Autodesk Inventor part; units mm, degrees
ref_plane "YZ Plane" through (0, 0, 0) normal (1, 0, 0) x (0, 1, 0)
ref_plane "XZ Plane" through (0, 0, 0) normal (0, 1, 0) x (-1, 0, 0)
ref_plane "XY Plane" through (0, 0, 0) normal (0, 0, 1) x (1, 0, 0)
sketch "Sketch1" plane through (0, 0, 0) normal (0, 1, 0) x (-1, 0, 0)
  circle A0 centre (0, 0) radius 7.5
  circle A1 centre (0, 0) radius 2.75
  dimension "d0" = 15
  dimension "d1" = 5.5
extrude "Extrusion1" add sketch "Sketch1" along normal blind 15
sketch "Sketch2" plane through (0, 15, 0) normal (0, 1, 0) x (1, 0, 0)
  circle A0 centre (0, 0) radius 2.75
  circle A1 centre (0, 0) radius 2.75
  circle A2 centre (0, 0) radius 4
  dimension "d4" = 5.5
  dimension "d5" = 8
extrude "Extrusion2" add sketch "Sketch2" along normal blind 5
fillet "Fillet1" radius 6.2 1 edges at (-4, 15, 0)
properties part number "Rollder_Spacer_Single"
The model under review builds one solid part; all positions refer to its coordinate system, in mm. Round coordinates to 2 decimals unless told otherwise and drop trailing zeros. Loops run counter-clockwise (first coordinate to the right, second up) from the corner with the lowest first, then second, coordinate; pieces in that order, holes last. Notation, with made-up numbers: (69, -5.75) -> (109, -5.75) arc R14 ccw to (109, 10.25) -> close; hole circle Ø9 at (-25.75, 65). An arc over 180 degrees is marked (long way). Return JSON: item names as keys, results as strings.
(1) Add section B-B on y = 3.25. Write out the cut boundary in (x, z).
Solved:
{"outline": "circle Ø15 at (0, 0); hole circle Ø5.5 at (0, 0)"}
(2) For pin 1 (3 mm diameter, centred on x = -5.5, y = 6.5, fed in from +Z); pin 2 (2 mm diameter, centred on y = 6, z = 4.5, fed in from +X); pin 3 (2 mm diameter, centred on x = -3.5, y = 9.5, fed in from +Z), all flat-tipped, find the tip position at first contact; note any pin that passes through.
Solved:
{"pin 1": "z = 6.34", "pin 2": "x = 6.63", "pin 3": "z = 7.07"}
(3) For line 1 (Z direction, x = 0, y = 4.75); line 2 (X direction, y = 15.75, z = 0), list the stretches that pass through material, from the lowest coordinate up.
Solved:
{"line 1": "-7.5 to -2.75, 2.75 to 7.5", "line 2": "-6.3 to -2.75, 2.75 to 6.3"}
